The listing builds one solid part. Answer for the finished solid, in the listing's coordinates (mm). A direction names the side the tool comes from. Give positions to 0.01 mm unless a question says otherwise; leave off trailing zeros. Order: outer loops, then holes, each group sorted by start corner. A loop starts at its lowest first (then second) coordinate and runs counter-clockwise, first axis right, second up. Notation, with made-up numbers: (60.25, 88) - (75.25, 88) arc R22 cw to (75.25, 115) - close; hole circle Ø4 at (-9, 7.5). An arc over 180 degrees is marked (long way). Use a Markdown table: item, result. Add a question column.
1) Find section C-C, the plane y = -1.25. Determine the outline of the cut face in (x, z).
2) Find section B-B, the plane y = -9.75. Determine the outline of the cut face in (x, z).
3) Find section A-A, the plane y = -6.5. Determine the outline of the cut face in (x, z), plus the area to 3 significant figures.
4) For faces 1 (the face through (-58, -10.607, 6)), 2 (the face through (-53.577, -8.881, 5.916)), 3 (the face through (-21.63, -9.57, 5.29)), determine the directions among +Z, -Z, +X, -X, +Y, -Y from which every point of the face is accessible in a straight line to the end or side of a thin tool.
5) The mould has two halves that part along X. Classify faces 4 (the face through (-25, -7.106, 2)), 5 (the face through (5, -5, 6)), 6 (the face through (-25, -4, 0)): released by +X, released by -X, zero draft, split by the parting line, or undercut.
6) Flat-ended cylindrical pins translate along their axes: pin 1 (5 mm diameter, centred on x = -6.5, z = 6, fed in from +Y); pin 2 (1 mm diameter, centred on y = -8.5, z = 10, fed in from +X); pin 3 (2 mm diameter, centred on x = -26, y = -10, fed in from +Z); pin 4 (6 mm diameter, centred on x = 8.5, z = 6.5, fed in from -Y). Find the tip coordinate at first contact, or state that the pin passes through.
7) Find section D-D, the plane x = -9. Determine the outline of the cut face in (y, z), plus the area to 3 significant figures.
8) Straight lines are drawn through the part: line 1 (Y direction, x = -35, z = 5.5); line 2 (X direction, y = -4.75, z = 5.5); line 3 (X direction, y = -3.25, z = 4.75). For each, find the intervals that lie inside material, in ascending order.
from build123d import *

# Parameters (mm, degrees)
Y_KSEKLIK_EKSTR_ZYON1_DEPTH = 12
KES_EKSTR_ZYON1_DEPTH       = 12
IZIM3_R                     = 3.451970481
Y_KSEKLIK_EKSTR_ZYON2_DEPTH = 5


with BuildPart() as part:
    # Çizim1 → Yükseklik-Ekstrüzyon1 (new body)
    with BuildSketch(Plane.XY):
        Polygon((0, 0), (-50, 0), (-60.606601718, -10.606601718), (-55.303300859, -10.606601718), (-51.802447925, -7.105748784), (1.802447925, -7.105748784), (5.303300859, -10.606601718), (10.606601718, -10.606601718), align=None)
    extrude(amount=Y_KSEKLIK_EKSTR_ZYON1_DEPTH)

    # Çizim2 → Kes-Ekstrüzyon1 (cut)
    with BuildSketch(Plane.XZ.offset(7.105748784)):
        with BuildLine():
            ThreePointArc((-23.536228909, 6.327680015), (-25, 7.5), (-26.463771091, 6.327680015))
            Line((-26.463771091, 6.327680015), (-25, 6))
            Line((-25, 6), (-23.536228909, 6.327680015))
        make_face()
        with BuildLine():
            Line((-25, 6), (-26.463771091, 6.327680015))
            ThreePointArc((-26.463771091, 6.327680015), (-26.5, 6), (-26.463771091, 5.672319985))
            Line((-26.463771091, 5.672319985), (-25, 6))
        make_face()
        with BuildLine():
            ThreePointArc((-23.5, 6), (-23.509084738, 6.16483835), (-23.536228909, 6.327680015))
            Line((-23.536228909, 6.327680015), (-25, 6))
            Line((-25, 6), (-23.536228909, 5.672319985))
            ThreePointArc((-23.536228909, 5.672319985), (-23.509084738, 5.83516165), (-23.5, 6))
        make_face()
        with BuildLine():
            Line((-25, 6), (-26.463771091, 5.672319985))
            ThreePointArc((-26.463771091, 5.672319985), (-25, 4.5), (-23.536228909, 5.672319985))
            Line((-23.536228909, 5.672319985), (-25, 6))
        make_face()
    extrude(amount=-KES_EKSTR_ZYON1_DEPTH, mode=Mode.SUBTRACT)

    # Çizim3 → Yükseklik-Ekstrüzyon2 (add)
    with BuildSketch(Plane.XZ.offset(7.105748784)):
        with Locations(Location((-25.000905718, 6.034003848, 0), (0, 0, 90))):
            Circle(IZIM3_R)
        with BuildLine():
            ThreePointArc((-23.572219211, 5.475380836), (-23.599693794, 5.409656229), (-23.630190025, 5.345277999))
            ThreePointArc((-23.630190025, 5.345277999), (-26.493538373, 6.387914237), (-23.46688981, 6.034003848))
            ThreePointArc((-23.46688981, 6.034003848), (-23.493452131, 5.74977069), (-23.572219211, 5.475380836))
        make_face(mode=Mode.SUBTRACT)
    extrude(amount=Y_KSEKLIK_EKSTR_ZYON2_DEPTH)


solid = part.part
The answers:
| question | item | result |
|---|---|---|
| 1 | outline | (-51.25, 0) - (1.25, 0) - (1.25, 12) - (-51.25, 12) - close; hole circle Ø3 at (-25, 6) |
| 2 | outline | (-59.75, 0) - (-54.45, 0) - (-54.45, 12) - (-59.75, 12) - close; circle Ø6.9 at (-25, 6.03); (4.45, 0) - (9.75, 0) - (9.75, 12) - (4.45, 12) - close; hole circle Ø3.07 at (-25, 6.03) |
| 3 | outline | (-56.5, 0) - (6.5, 0) - (6.5, 12) - (-56.5, 12) - close; hole circle Ø3 at (-25, 6) |
| 3 | area | 749 mm2 |
| 4 | face 1 | +Z, -Z, -X, -Y |
| 4 | face 2 | +Z, -Z, -Y |
| 4 | face 3 | -Y |
| 5 | face 4 | undercut |
| 5 | face 5 | released by +X |
| 5 | face 6 | zero draft |
| 6 | pin 1 | y = 0 |
| 6 | pin 2 | x = 9 |
| 6 | pin 3 | z = 9.49 |
| 6 | pin 4 | y = -10.61 |
| 7 | outline | (-7.11, 0) - (0, 0) - (0, 12) - (-7.11, 12) - close |
| 7 | area | 85.3 mm2 |
| 8 | line 1 | -7.11 to 0 |
| 8 | line 2 | -54.75 to -26.41, -23.59 to 4.75 |
| 8 | line 3 | -53.25 to -25.83, -24.17 to 3.25 |
